For this review, take the finished solid that the model builds, in its own axes (mm). A direction names the side the tool comes from. Give positions to 0.01 mm unless a question says otherwise; leave off trailing zeros. Loops run counter-clockwise (first coordinate to the right, second up) from the corner with the lowest first, then second, coordinate; pieces in that order, holes last. Notation, with made-up numbers: (69.25, -28) - (87.25, -28) arc R25 ccw to (87.25, -5) - close; hole circle Ø1 at (46, 66). An arc over 180 degrees is marked (long way). Answer as CSV lines item,"result".
from build123d import *

# Parameters (mm, degrees)
SKETCH_1_W          = 15
SKETCH_1_H          = 15
SKETCH_1_W_2        = 12
SKETCH_1_H_2        = 12
EXTRUDE_1_DEPTH     = 240
SKETCH_2_R          = 1.6
CUT_EXTRUDE_1_DEPTH = 241.585223985
SKETCH_3_R          = 1.6
CUT_EXTRUDE_2_DEPTH = 241.585223985


with BuildPart() as part:
    # ｽｹｯﾁ1 → ﾎﾞｽ - 押し出し1 (new body)
    with BuildSketch(Plane.XY):
        Rectangle(SKETCH_1_W, SKETCH_1_H)
        Rectangle(SKETCH_1_W_2, SKETCH_1_H_2, mode=Mode.SUBTRACT)
    extrude(amount=EXTRUDE_1_DEPTH)

    # ｽｹｯﾁ2 → ｶｯﾄ - 押し出し1 (cut, through all)
    with BuildSketch(Plane(origin=(0, 7.5, 0), x_dir=(1, 0, 0), z_dir=(0, 1, 0))):
        with Locations(Location((0, -22.5, 0), (0, 0, 270))):
            Circle(SKETCH_2_R)
        with Locations(Location((0, -217.5, 0), (0, 0, 270))):
            Circle(SKETCH_2_R)
    extrude(amount=-CUT_EXTRUDE_1_DEPTH, mode=Mode.SUBTRACT)

    # ｽｹｯﾁ3 → ｶｯﾄ - 押し出し2 (cut, through all)
    with BuildSketch(Plane(origin=(7.5, 0, 0), x_dir=(0, 0, -1), z_dir=(1, 0, 0))):
        with Locations((-232.5, 0)):
            Circle(SKETCH_3_R)
        with Locations((-7.5, 0)):
            Circle(SKETCH_3_R)
    extrude(amount=-CUT_EXTRUDE_2_DEPTH, mode=Mode.SUBTRACT)


solid = part.part
1) Wall thickness on line 1 (X direction, y = -6.75, z = 22.5); line 2 (X direction, y = 5.75, z = 215.5): over which ranges is each line inside the solid? List them lowest first. Write a range as from..to.
From the geometry:
line 1,"x = -7.5..-1.6, 1.6..7.5"
line 2,"x = -7.5..-6, 6..7.5"
2) Consider section A-A on z = 206. Write out the cut boundary in (x, y), and give its area (3 significant figures).
From the geometry:
outline,"(-7.5, -7.5) - (7.5, -7.5) - (7.5, 7.5) - (-7.5, 7.5) - close; hole (-6, -6) - (6, -6) - (6, 6) - (-6, 6) - close"
area,"81.0 mm^2"
3) Machinability: for faces 4 (the flat face through (0, -6, 118)), 5 (the flat face through (7.5, 0, 118)), which of the approach directions +Z, -Z, +X, -X, +Y, -Y give a long, thin tool a straight path to every point of the face, cutting with its end or side? Answer none if there is none.
From the geometry:
face 4,"+Z, -Z"
face 5,"+Z, -Z, +X, +Y, -Y"
4) Draft analysis for pull direction Y (two halves, no side actions). For faces 1 (the flat face through (0, 6, 118)), 2 (the flat face through (0, -7.5, 118)), 3 (the flat face through (-7, 0, 240)), state which applies: pulls with the +Y half, pulls with the -Y half, needs draft (parallel to the pull), parting line crosses it, or undercut.
From the geometry:
face 1,"undercut"
face 2,"pulls with the -Y half"
face 3,"needs draft"
